```python
from build123d import *

# Parameters (mm, degrees)
F1_DEPTH = 500
F3_DEPTH = 60.001
F4_R     = 4.5
F5_DEPTH = 60.001


with BuildPart() as f1:
    # F0 (on Front) → F1 (new body)
    with BuildSketch(Plane.XZ):
        Polygon((60, 0), (0, 0), (0, -60), (2.5, -60), (2.5, -2.5), (60, -2.5), align=None)
    extrude(amount=F1_DEPTH)

    # F2 (on face) → F3 (cut, through all)
    with BuildSketch(Plane(origin=(0, 0, 0), x_dir=(0, -1, 0), z_dir=(-1, 0, 0))):
        Polygon((500, -60), (500, 0), (440, -60), align=None)
    extrude(amount=-F3_DEPTH, mode=Mode.SUBTRACT)

    # F4 (on face) → F5 (cut, through all)
    with BuildSketch(Plane.XY):
        with Locations((30, -100)):
            Circle(F4_R)
        with Locations((30, -200)):
            Circle(F4_R)
        with Locations((30, -300)):
            Circle(F4_R)
        with Locations((30, -400)):
            Circle(F4_R)
    extrude(amount=-F5_DEPTH, mode=Mode.SUBTRACT)


solid = f1.part
```
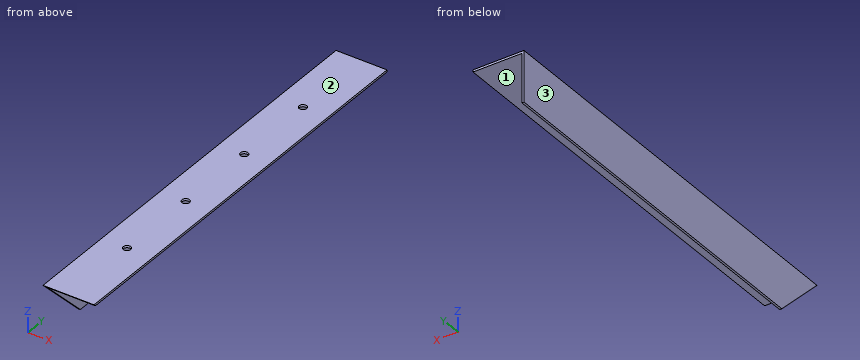
Work out the finished part from the listing and answer in its coordinate system (mm). Face numbers are marked on the shaded views. Round coordinates to 2 decimals unless told otherwise and drop trailing zeros. Loops run counter-clockwise (first coordinate to the right, second up) from the corner with the lowest first, then second, coordinate; pieces in that order, holes last. Notation, with made-up numbers: M 69.5,26 L 88.5,26 A18 cw 88.5,36 Z; hole C 57.5,-9.5 d9. An arc over 180 degrees is marked long. Use CSV: the item, a comma, the result in double quotes.
Q1. Section B-B, the plane y = -400 is taken. Determine the outline of the cut face in (x, z).
Determined:
outline,"M 0,-60 L 2.5,-60 L 2.5,-2.5 L 25.5,-2.5 L 25.5,0 L 0,0 Z; M 34.5,-2.5 L 60,-2.5 L 60,0 L 34.5,0 Z"
Q2. Section C-C, the plane y = -468.5 is taken. Determine the outline of the cut face in (x, z).
Determined:
outline,"M 0,-31.5 L 2.5,-31.5 L 2.5,-2.5 L 60,-2.5 L 60,0 L 0,0 Z"
Q3. Section A-A, the plane x = 30 is taken. Determine the outline of the cut face in (y, z), then the cut area to 3 significant figures.
Determined:
outline,"M -500,0 L -497.5,-2.5 L -404.5,-2.5 L -404.5,0 Z; M -395.5,-2.5 L -304.5,-2.5 L -304.5,0 L -395.5,0 Z; M -295.5,-2.5 L -204.5,-2.5 L -204.5,0 L -295.5,0 Z; M -195.5,-2.5 L -104.5,-2.5 L -104.5,0 L -195.5,0 Z; M -95.5,-2.5 L 0,-2.5 L 0,0 L -95.5,0 Z"
area,"1,160 mm2"
Q4. Consider L1, parallel to X at y = -300, z = -1.85; L2, parallel to Z at x = 28, y = -365.5; L3, parallel to Y at x = 30, z = -1.1. Determine where each line is inside the solid, lowest interval first.
Determined:
L1,"0 to 25.5, 34.5 to 60"
L2,"-2.5 to 0"
L3,"-498.9 to -404.5, -395.5 to -304.5, -295.5 to -204.5, -195.5 to -104.5, -95.5 to 0"
Q5. Section D-D, the plane z = -8 is taken. Determine the outline of the cut face in (x, y).
Determined:
outline,"M 0,-492 L 2.5,-492 L 2.5,0 L 0,0 Z"
Q6. Each of these flat-tipped pins is pushed along its axis until it touches: pin 1 (6 mm diameter, centred on y = -260, z = -43, fed in from -X); pin 2 (1.5 mm diameter, centred on x = 14, y = -166.5, fed in from -Z); pin 3 (5 mm diameter, centred on y = -329.5, z = -46.5, fed in from +X). Where does it stop, or does it pass through?
Determined:
pin 1,"x = 0"
pin 2,"z = -2.5"
pin 3,"x = 2.5"
Q7. The mould has two halves that part along Z. Classify the marked faces 1, 2 and 3: pulls with the +Z half, pulls with the -Z half, needs draft (parallel to the pull), parting line crosses it, or undercut.
Determined:
face 1,"pulls with the -Z half"
face 2,"pulls with the +Z half"
face 3,"needs draft"
